Geometry check sheet. Reference: the model listing, model coordinates, mm. A direction names the side the tool comes from. Round coordinates to 2 decimals unless told otherwise and drop trailing zeros. Write each loop counter-clockwise with the first axis right and the second up, starting at its lowest first coordinate (ties: lowest second). Pieces come first, ordered by that corner, then holes. Notation, with made-up numbers: (0.25, 65.5) -> (41.25, 65.5) arc R31 ccw to (41.25, 89.5) -> close; hole circle Ø6 at (34.25, -2). An arc over 180 degrees is marked (long way). Use a Markdown table: item, result.
```python
from build123d import *

# Parameters (mm, degrees)
F0_W     = 127
F0_H     = 63.5
F1_DEPTH = 38.1
F3_DEPTH = 50.8
F5_DEPTH = 19.05


with BuildPart() as f1:
    # F0 (on Front) → F1 (new body)
    with BuildSketch(Plane.XZ):
        with Locations((5.649563, -19.189008)):
            Rectangle(F0_W, F0_H)
    extrude(amount=F1_DEPTH)

    # F2 (on Front) → F3 (cut)
    with BuildSketch(Plane.XZ):
        Polygon((-57.850437, -12.839008), (-32.450437, 12.560992), (-61.992485, 12.560992), (-61.992485, -12.82603), align=None)
    extrude(amount=F3_DEPTH, mode=Mode.SUBTRACT)

    # F4 (on Front) → F5 (cut)
    with BuildSketch(Plane.XZ):
        Polygon((-19.750437, -50.939008), (43.749563, 12.560992), (-59.24404, 12.560992), (-59.24404, -50.99874), align=None)
    extrude(amount=F5_DEPTH, mode=Mode.SUBTRACT)


solid = f1.part
```
(1) Access from +Z, -Z, +X, -X, +Y, -Y to the whole of each face (thin tool, end or side, straight path). Record for faces 1 (the face through (-19, -19.05, -19)), 2 (the face through (-57.85, -28, -32)).
A:
| item | result |
|---|---|
| face 1 | +Z, -X, +Y |
| face 2 | +Z, -Z, -X, +Y, -Y |
(2) Section check A-A on y = -35. Record the cut outline in (x, z).
A:
| item | result |
|---|---|
| outline | (-57.85, -50.94) -> (69.15, -50.94) -> (69.15, 12.56) -> (-32.45, 12.56) -> (-57.85, -12.84) -> close |
(3) Thickness scan on line 1 (Y direction, x = -34, z = -30); line 2 (X direction, y = -32, z = -4); line 3 (X direction, y = -19, z = -1). Record the ranges inside material, lowest first.
A:
| item | result |
|---|---|
| line 1 | y = -38.1 to -19.05 |
| line 2 | x = -49.01 to 69.15 |
| line 3 | x = 30.19 to 69.15 |
(4) Gauge pin test, flat ends, axial feed: pin 1 Ø2 at (x, z) = (14, 0.5) entering from +Y; pin 2 Ø10 at (x, z) = (47.5, 2) entering from +Y. Record the tip position at first contact, or that the pin passes through.
A:
| item | result |
|---|---|
| pin 1 | stops at y = -19.05 |
| pin 2 | stops at y = 0 |
(5) Section check C-C on z = -30.5. Record the cut outline in (x, y).
A:
| item | result |
|---|---|
| outline | (-57.85, -38.1) -> (69.15, -38.1) -> (69.15, 0) -> (0.69, 0) -> (0.69, -19.05) -> (-57.85, -19.05) -> close |
(6) Section check D-D on y = -12. Record the cut outline in (x, z), plus the area to 3 significant figures.
A:
| item | result |
|---|---|
| outline | (-19.75, -50.94) -> (69.15, -50.94) -> (69.15, 12.56) -> (43.75, 12.56) -> close |
| area | 3,630 mm2 |
(7) Section check B-B on x = 10. Record the cut outline in (y, z), plus the area to 3 significant figures.
A:
| item | result |
|---|---|
| outline | (-38.1, -50.94) -> (0, -50.94) -> (0, -21.19) -> (-19.05, -21.19) -> (-19.05, 12.56) -> (-38.1, 12.56) -> close |
| area | 1,780 mm2 |
